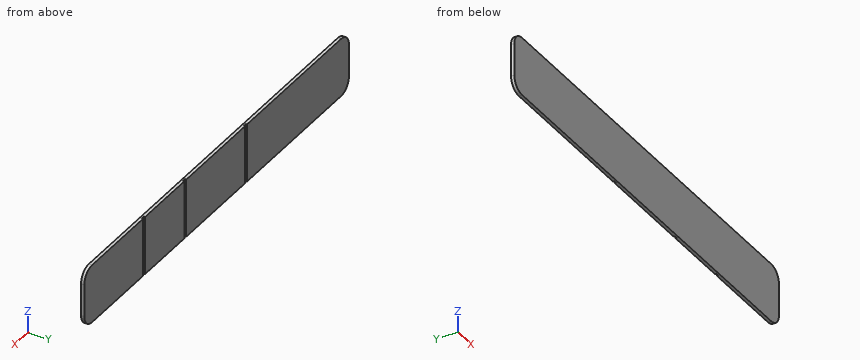
```python
from build123d import *

# Parameters (mm, degrees)
SKETCH1_W           = 135
SKETCH1_H           = 18
BOSS_EXTRUDE1_DEPTH = 1
SKETCH2_W           = 1
SKETCH2_H           = 18
CUT_EXTRUDE1_DEPTH  = 0.4
FILLET1_R           = 4


with BuildPart() as part:
    # Sketch1 → Boss-Extrude1 (new body)
    with BuildSketch(Plane(origin=(0, 0, 0), x_dir=(1, 0, 0), z_dir=(0, 1, 0))):
        with Locations((67.5, 9)):
            Rectangle(SKETCH1_W, SKETCH1_H)
    extrude(amount=BOSS_EXTRUDE1_DEPTH)

    # Sketch2 → Cut-Extrude1 (cut)
    with BuildSketch(Plane(origin=(0, 1, 0), x_dir=(1, 0, 0), z_dir=(0, 1, 0))):
        with Locations((52.5, 9)):
            Rectangle(SKETCH2_W, SKETCH2_H)
        with Locations((83.5, 9)):
            Rectangle(SKETCH2_W, SKETCH2_H)
        with Locations((104.5, 9)):
            Rectangle(SKETCH2_W, SKETCH2_H)
    extrude(amount=-CUT_EXTRUDE1_DEPTH, mode=Mode.SUBTRACT)

    # Fillet1
    fillet1_edges = [part.edges().sort_by_distance(p)[0] for p in [
        (0, 0.5, 0),
        (0, 0.5, -18),
        (135, 0.5, -18),
        (135, 0.5, 0),
    ]]
    fillet(fillet1_edges, radius=FILLET1_R)


solid = part.part
```
Work out the finished part from the listing and answer in its coordinate system (mm). Round coordinates to 2 decimals unless told otherwise and drop trailing zeros. Write each loop counter-clockwise with the first axis right and the second up, starting at its lowest first coordinate (ties: lowest second). Pieces come first, ordered by that corner, then holes. Notation, with made-up numbers: (-27, -2) - (29, -2) arc R24 cw to (29, 12) - close; hole circle Ø5 at (59.25, 30.5). An arc over 180 degrees is marked (long way). Return JSON: item names as keys, results as strings. Group by question number.
Q1. The part is cut by section B-B on z = -16. Write down the section's boundary in (x, y), then the cut area to 3 significant figures.
Q2. The part is cut by section A-A on y = 0.85. Write down the section's boundary in (x, z), then the cut area to 3 significant figures.
Q3. Each of these flat-tipped pins is pushed along its axis until it touches: pin 1 Ø8 at (x, z) = (84, -2.5) entering from -Y; pin 2 Ø0.8 at (x, z) = (104.5, -12.5) entering from +Y. Where does it stop, or does it pass through?
Q4. Find the intervals of material crossed by L1, parallel to X at y = 0.65, z = -9.5; L2, parallel to X at y = 0.4, z = -3.75; L3, parallel to X at y = 0.2, z = -17, in increasing order.
Solved:
{
 "1": {"outline": "(0.54, 0) - (134.46, 0) - (134.46, 1) - (105, 1) - (105, 0.6) - (104, 0.6) - (104, 1) - (84, 1) - (84, 0.6) - (83, 0.6) - (83, 1) - (53, 1) - (53, 0.6) - (52, 0.6) - (52, 1) - (0.54, 1) - close", "area": "133 mm²"},
 "2": {"outline": "(0, -14) arc R4 ccw to (4, -18) - (52, -18) - (52, 0) - (4, 0) arc R4 ccw to (0, -4) - close; (53, -18) - (83, -18) - (83, 0) - (53, 0) - close; (84, -18) - (104, -18) - (104, 0) - (84, 0) - close; (105, -18) - (131, -18) arc R4 ccw to (135, -14) - (135, -4) arc R4 ccw to (131, 0) - (105, 0) - close", "area": "2,360 mm²"},
 "3": {"pin 1": "y = 0", "pin 2": "y = 0.6"},
 "4": {"L1": "0 to 52, 53 to 83, 84 to 104, 105 to 135", "L2": "0.01 to 134.99", "L3": "1.35 to 133.65"}
}
